Job drawing, mm, ordinate dimensions from the low corner. One solid piece. A direction names the side the tool comes from. Give positions to 0.01 mm unless a question says otherwise; leave off trailing zeros. Write each loop counter-clockwise with the first axis right and the second up, starting at its lowest first coordinate (ties: lowest second). Pieces come first, ordered by that corner, then holes. Notation, with made-up numbers: M -31,70.25 L -13,70.25 A29 cw -13,107.25 Z; hole C -22,-7 d11. An arc over 180 degrees is marked long. Answer as CSV lines item,"result". Start each with the question number.
Item 1: Band-saw the part on D-D, the plane x = 7. List the corners of the cut face in (y, z).
Item 2: Two-plate mould, pull along Z, no slides. Class the marked faces 1, 2, 3 and 4: +Z half, -Z half, draft (parallel to the pull), parting line (faces both ways), or undercut.
Item 3: Band-saw the part on C-C, the plane y = 0.65. List the corners of the cut face in (x, z) (1 decimal), then the cut area to 3 significant figures.
Item 4: Wall check: L1, parallel to Y at x = 5, z = 7.25; L2, parallel to Z at x = 8.75, y = 2.6 (1 decimal); L3, parallel to X at y = 2.7, z = 12.25. Give the ranges that are in metal, low to high. Write a range as from..to.
Item 5: 3-axis set-ups, long thin cutter, end or side, ignore diameter. For the marked faces 5 and 6: which of +Z, -Z, +X, -X, +Y, -Y reach the whole face in a straight line?
Item 6: Pin check, flat tips, straight feed: pin 1 (2 mm diameter, centred on y = 4.5, z = 9, fed in from +X); pin 2 (5.5 mm diameter, centred on x = 10.98, z = 10.98, fed in from -Y); pin 3 (3 mm diameter, centred on x = 3.63, z = 10.98, fed in from +Y). Stop position of each tip, or through.
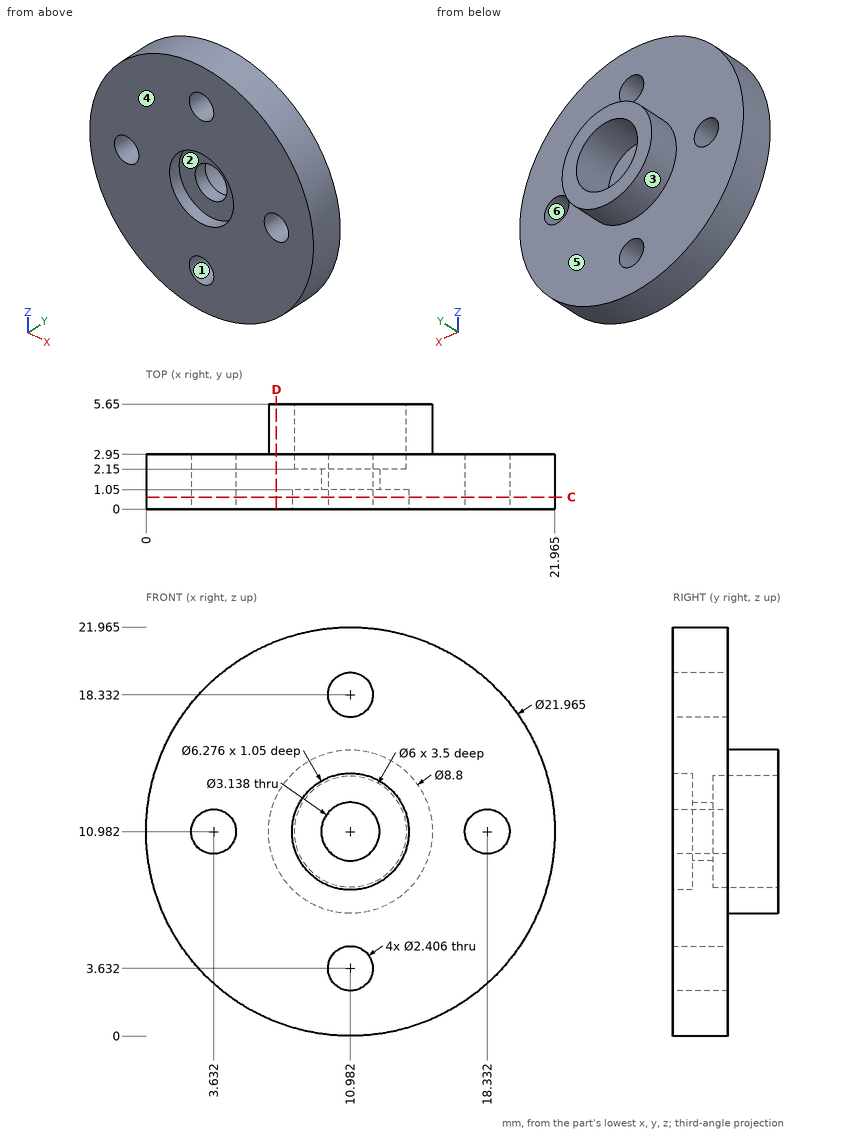
Output:
1,outline,"M 0,0.75 L 2.95,0.75 L 2.95,9.11 L 5.65,9.11 L 5.65,12.85 L 2.95,12.85 L 2.95,21.22 L 0,21.22 Z"
2,face 1,"undercut"
2,face 2,"undercut"
2,face 3,"parting line"
2,face 4,"draft"
3,outline,"C 11,11 d22; hole C 3.6,11 d2.4; hole C 11,11 d6.3; hole C 11,3.6 d2.4; hole C 11,18.3 d2.4; hole C 18.3,11 d2.4"
3,area,"330 mm²"
4,L1,"0..2.95"
4,L2,"0.2..9, 13..21.7"
4,L3,"0.07..8.26, 13.7..21.89"
5,face 5,"+Y"
5,face 6,"+Y, -Y"
6,pin 1,"x = 15.27"
6,pin 2,"y = 1.05"
6,pin 3,"y = 2.95"
